Part model, mm, in its own coordinate system. Give positions to 0.01 mm unless a question says otherwise; leave off trailing zeros. Write each loop counter-clockwise with the first axis right and the second up, starting at its lowest first coordinate (ties: lowest second). Pieces come first, ordered by that corner, then holes. Notation, with made-up numbers: M -34.75,48.25 L -26.75,48.25 A21 ccw -26.75,65.25 Z; hole C -34,4 d8. An arc over 180 degrees is marked long. Use CSV: the item, a comma, the result in double quotes. Start each with the question number.
Item 1: Drill centre lines: line 1 (Z direction, x = -7, y = -1); line 2 (Y direction, x = 4.25, z = 112.5). Where is each one in solid material? Low to high. Write a range as [from, to].
Item 2: Cut at A-A (z = 265). List the corners of the cut face in (x, y), then the cut area to 3 significant figures.
Item 3: Pin check, flat tip, straight feed: pin 1 (9 mm diameter, centred on x = 0, z = 42.5, fed in from -Y). Stop position of the tip, or through.
Item 4: Cut at B-B (y = 0). Count the separate pieces of the cut face and the enclosed holes in it, then the cut area to 3 significant figures.
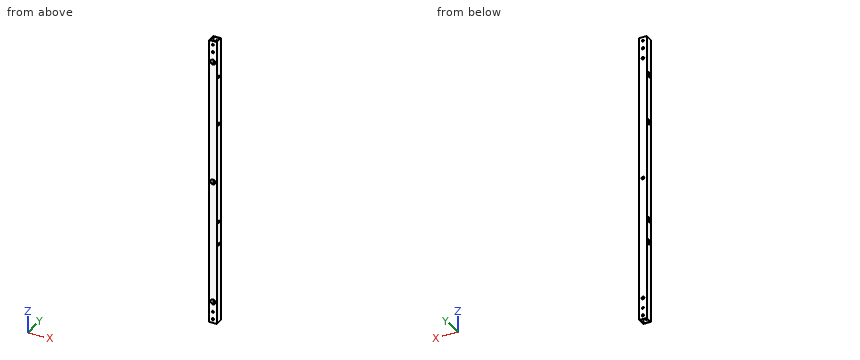
from build123d import *

# Parameters (mm, degrees)
SKETCH_1_W                  = 15
SKETCH_1_H                  = 15
SKETCH_1_W_2                = 12
SKETCH_1_H_2                = 12
EXTRUDE_1_DEPTH             = 568
SKETCH_5_R                  = 2
SKETCH_5_R_2                = 2.25
SKETCH_5_R_3                = 2.7
CUT_EXTRUDE_4_DEPTH         = 20
SKETCH_9_R                  = 2.7
CUT_EXTRUDE_6_DEPTH         = 40
SKETCH_10_R                 = 5
CUT_EXTRUDE_7_DEPTH         = 5
HOLE_WIZARD_10_0_10_2_D     = 10
HOLE_WIZARD_10_0_10_2_DEPTH = 1.5


with BuildPart() as part:
    # ｽｹｯﾁ1 → ﾎﾞｽ - 押し出し1 (new body)
    with BuildSketch(Plane.XY):
        Rectangle(SKETCH_1_W, SKETCH_1_H)
        Rectangle(SKETCH_1_W_2, SKETCH_1_H_2, mode=Mode.SUBTRACT)
    extrude(amount=EXTRUDE_1_DEPTH)

    # ｽｹｯﾁ5 → ｶｯﾄ - 押し出し4 (cut)
    with BuildSketch(Plane(origin=(0, -7.5, 0), x_dir=(-1, 0, 0), z_dir=(0, -1, 0))):
        with Locations((0, -22.5)):
            Circle(SKETCH_5_R)
        with Locations((0, -7.5)):
            Circle(SKETCH_5_R_2)
        with Locations((0, -560.5)):
            Circle(SKETCH_5_R)
        with Locations((0, -545.5)):
            Circle(SKETCH_5_R_2)
        with Locations((0, -42.5)):
            Circle(SKETCH_5_R_3)
        with Locations((0, -284)):
            Circle(SKETCH_5_R_3)
        with Locations((0, -525.5)):
            Circle(SKETCH_5_R_3)
    extrude(amount=-CUT_EXTRUDE_4_DEPTH, mode=Mode.SUBTRACT)

    # ｽｹｯﾁ9 → ｶｯﾄ - 押し出し6 (cut)
    with BuildSketch(Plane(origin=(7.5, 0, 0), x_dir=(0, 0, -1), z_dir=(1, 0, 0))):
        with Locations((-494, 0)):
            Circle(SKETCH_9_R)
        with Locations((-399, 0)):
            Circle(SKETCH_9_R)
        with Locations((-202, 0)):
            Circle(SKETCH_9_R)
        with Locations((-157, 0)):
            Circle(SKETCH_9_R)
    extrude(amount=-CUT_EXTRUDE_6_DEPTH, mode=Mode.SUBTRACT)

    # ｽｹｯﾁ10 → ｶｯﾄ - 押し出し7 (cut)
    with BuildSketch(Plane.ZY.offset(7.5)):
        with Locations((157, 0)):
            Circle(SKETCH_10_R)
        with Locations((202, 0)):
            Circle(SKETCH_10_R)
        with Locations((399, 0)):
            Circle(SKETCH_10_R)
        with Locations((494, 0)):
            Circle(SKETCH_10_R)
    extrude(amount=-CUT_EXTRUDE_7_DEPTH, mode=Mode.SUBTRACT)

    # Ø10.0 (10) 直径の穴2
    with Locations(Plane(origin=(0, -7.5, 0), x_dir=(-1, 0, 0), z_dir=(0, -1, 0))):
        with Locations((0, -42.5), (0, -284), (0, -525.5)):
            Hole(HOLE_WIZARD_10_0_10_2_D / 2, depth=HOLE_WIZARD_10_0_10_2_DEPTH)


solid = part.part
Worked answers:
1,line 1,"z = [0, 152.1], [161.9, 197.1], [206.9, 394.1], [403.9, 489.1], [498.9, 568]"
1,line 2,"y = [-7.5, -6], [6, 7.5]"
2,outline,"M -7.5,-7.5 L 7.5,-7.5 L 7.5,7.5 L -7.5,7.5 Z; hole M -6,-6 L 6,-6 L 6,6 L -6,6 Z"
2,area,"81.0 mm^2"
3,pin 1,"stops at y = 6"
4,separate pieces,"10"
4,enclosed holes,"0"
4,area,"1,610 mm^2"
